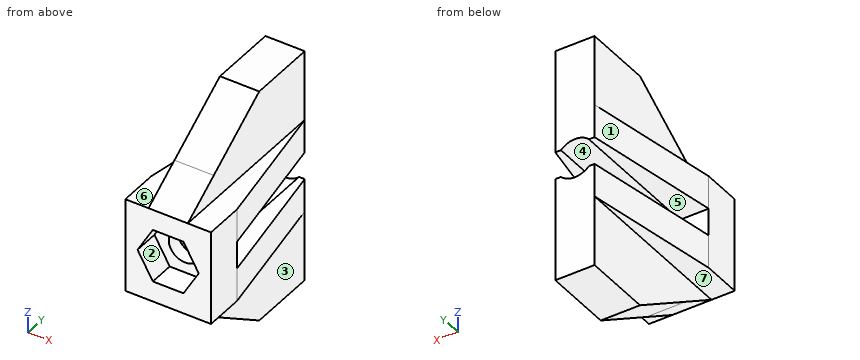
```python
from build123d import *

# Parameters (mm, degrees)
SKETCH1_W           = 21.82
SKETCH1_H           = 24
SKETCH1_R           = 4.15
BOSS_EXTRUDE1_DEPTH = 5
CUT_EXTRUDE1_DEPTH  = 6.5
BOSS_EXTRUDE2_DEPTH = 35
BOSS_EXTRUDE3_DEPTH = 10
CUT_EXTRUDE2_DEPTH  = 10
BOSS_EXTRUDE4_START = -18
BOSS_EXTRUDE4_DEPTH = 8.5


with BuildPart() as part:
    # Sketch1 → Boss-Extrude1 (new, symmetric)
    with BuildSketch(Plane(origin=(0, 0, 0), x_dir=(1, 0, 0), z_dir=(0, 1, 0))):
        Rectangle(SKETCH1_W, SKETCH1_H)
        with Locations(Location((0, 0, 0), (0, 0, 270))):
            Circle(SKETCH1_R, mode=Mode.SUBTRACT)
    extrude(amount=BOSS_EXTRUDE1_DEPTH, both=True)

    # Sketch2 → Cut-Extrude1 (cut)
    with BuildSketch(Plane.XZ.offset(5)):
        Polygon((-7.794228634, 0), (-3.897114317, -6.75), (3.897114317, -6.75), (7.794228634, 0), (3.897114317, 6.75), (-3.897114317, 6.75), align=None)
    extrude(amount=-CUT_EXTRUDE1_DEPTH, mode=Mode.SUBTRACT)

    # Sketch3 → Boss-Extrude2 (add)
    with BuildSketch(Plane(origin=(0, 5, 0), x_dir=(1, 0, 0), z_dir=(0, 1, 0))):
        with BuildLine():
            Line((-3.570714214, 3.5), (-5, 3.5))
            Line((-5, 3.5), (-5, 30))
            Line((-5, 30), (5, 30))
            Line((5, 30), (5, 3.5))
            Line((5, 3.5), (3.570714214, 3.5))
            ThreePointArc((3.570714214, 3.5), (0, 5), (-3.570714214, 3.5))
        make_face()
        with BuildLine():
            Line((-5, -30), (5, -30))
            Line((5, -30), (5, -3.5))
            Line((5, -3.5), (3.570714214, -3.5))
            ThreePointArc((3.570714214, -3.5), (0, -5), (-3.570714214, -3.5))
            Line((-3.570714214, -3.5), (-5, -3.5))
            Line((-5, -3.5), (-5, -30))
        make_face()
    extrude(amount=BOSS_EXTRUDE2_DEPTH)

    # Sketch4 → Boss-Extrude3 (add)
    with BuildSketch(Plane(origin=(5, 0, 0), x_dir=(0, 0, -1), z_dir=(1, 0, 0))):
        Polygon((-10.166411733, -5), (-10.1597678, 5.000488901), (-30, 22.5), (-12, -5), align=None)
        Polygon((10.166411733, -5), (10.1597678, 5.000488901), (30, 22.5), (12, -5), align=None)
    extrude(amount=-BOSS_EXTRUDE3_DEPTH)

    # Sketch5 → Cut-Extrude2 (cut)
    with BuildSketch(Plane(origin=(5, 0, 0), x_dir=(0, 0, -1), z_dir=(1, 0, 0))):
        Polygon((-18.545454545, 5), (-30, 22.5), (-30, 5), align=None)
        Polygon((30, 22.5), (30, 5), (18.545454545, 5), align=None)
    extrude(amount=-CUT_EXTRUDE2_DEPTH, mode=Mode.SUBTRACT)

    # Sketch6 → Boss-Extrude4 (add)
    with BuildSketch(Plane(origin=(0, 0, -30), x_dir=(-1, 0, 0), z_dir=(0, 0, -1)).offset(BOSS_EXTRUDE4_START)):
        Polygon((-10.91, 5), (-5, 40), (-5, 5), align=None)
        Polygon((5, 40), (5, 5), (10.91, 5), align=None)
    boss_extrude4 = extrude(amount=-BOSS_EXTRUDE4_DEPTH)

    # Mirror9: Boss-Extrude4 across plane
    add(boss_extrude4.mirror(Plane.XY))


solid = part.part
```
Model file for the job. Use its own axes, mm. Face numbers are marked on the shaded views. A direction names the side the tool comes from. Coordinates: 2 decimals unless noted, no trailing zeros. Loops run counter-clockwise (first coordinate to the right, second up) from the corner with the lowest first, then second, coordinate; pieces in that order, holes last. Notation, with made-up numbers: (85.5, 13.25) - (114.5, 13.25) arc R14 ccw to (114.5, 20.25) - close; hole circle Ø8 at (85.5, -25.5). An arc over 180 degrees is marked (long way). Write item = value, one per line. Start each with the question number.
Item 1: Wall check: probe 1 along X at (y, z) = (3.55, 0); probe 2 along Z at (x, y) = (0, 4.1); probe 3 along Z at (x, y) = (4, 11). Give the ranges that are in metal, low to high. Write a range as [from, to].
Item 2: Drop flat-ended pins along their axis: pin 1 Ø2 at (y, z) = (6.5, 17) entering from -X; pin 2 Ø2 at (x, y) = (8, 23.5) entering from -Z; pin 3 Ø8 at (x, y) = (-7.5, 25.5) entering from +Z; pin 4 Ø1.5 at (x, y) = (8.5, 13.5) entering from +Z. Give the stop position or say it passes through.
Item 3: Saw through at C-C, the plane z = -2. List the corners of the cut face in (x, y), then the cut area to 3 significant figures.
Item 4: Saw through at B-B, the plane y = 12.5. List the corners of the cut face in (x, z).
Item 5: 3-axis set-ups, long thin cutter, end or side, ignore diameter. For the marked faces 4, 5, 6 and 7: which of +Z, -Z, +X, -X, +Y, -Y reach the whole face in a straight line?
Item 6: Pull direction X, two halves, no side cores. Call the marked faces 1, 2 and 3: +X half, -X half, draft (parallel to the pull), parting line (faces both ways), or undercut.
Item 7: Saw through at A-A, the plane x = 0. List the corners of the cut face in (y, z).
Item 8: Saw through at D-D, the plane x = 8.5. List the corners of the cut face in (y, z), then the cut area to 3 significant figures.
Answers:
q1.probe_1 = [-10.91, -4.15], [4.15, 10.91]
q1.probe_2 = [-17.96, -4.15], [4.15, 17.96]
q1.probe_3 = [-22.47, -3.5], [3.5, 22.47]
q2.pin_1 = -5
q2.pin_2 = -12
q2.pin_3 = 30
q2.pin_4 = 12
q3.outline = (-10.91, -5) - (-6.64, -5) - (-6.64, 1.5) - (-3.64, 1.5) - (-3.64, 5) - (-10.91, 5) - close; (3.64, 1.5) - (6.64, 1.5) - (6.64, -5) - (10.91, -5) - (10.91, 5) - (3.64, 5) - close
q3.area = 106 mm2
q4.outline = (-9.64, -12) - (-5, -12) - (-5, -23.45) - (5, -23.45) - (5, -12) - (9.64, -12) - (9.64, -3.5) - (3.57, -3.5) arc R5 cw to (-3.57, -3.5) - (-9.64, -3.5) - close; (-9.64, 3.5) - (-3.57, 3.5) arc R5 cw to (3.57, 3.5) - (9.64, 3.5) - (9.64, 12) - (5, 12) - (5, 23.45) - (-5, 23.45) - (-5, 12) - (-9.64, 12) - close
q5.face_4 = +Y
q5.face_5 = +X, -X, +Y
q5.face_6 = +Z, -X, +Y, -Y
q5.face_7 = -Z, -X, +Y, -Y
q6.face_1 = -X half
q6.face_2 = undercut
q6.face_3 = +X half
q7.outline = (-5, -12) - (22.5, -30) - (40, -30) - (40, -5) - (5, -5) - (5, -4.15) - (1.5, -4.15) - (1.5, -6.75) - (-5, -6.75) - close; (-5, 6.75) - (1.5, 6.75) - (1.5, 4.15) - (5, 4.15) - (5, 5) - (40, 5) - (40, 30) - (22.5, 30) - (-5, 12) - close
q8.outline = (-5, -12) - (19.27, -12) - (19.27, -3.5) - (5, -3.5) - (5, 3.5) - (19.27, 3.5) - (19.27, 12) - (-5, 12) - close
q8.area = 483 mm2
